Could you check a few things on this model? Use its own coordinates, in mm. Face numbers are marked on the shaded views. A direction names the side the tool comes from. Give positions to 0.01 mm unless a question says otherwise; leave off trailing zeros. Order: outer loops, then holes, each group sorted by start corner. A loop starts at its lowest first (then second) coordinate and runs counter-clockwise, first axis right, second up. Notation, with made-up numbers: (77.5, -11.5) - (98.5, -11.5) arc R28 ccw to (98.5, 23.5) - close; hole circle Ø11 at (41, -2). An arc over 180 degrees is marked (long way). Put each result on its own line as item: value.
from build123d import *

# Parameters (mm, degrees)
SKETCH1_W           = 100
SKETCH1_H           = 50
BOSS_EXTRUDE1_DEPTH = 15
SKETCH2_W           = 100
SKETCH2_H           = 65
BOSS_EXTRUDE2_DEPTH = 46
CUT_EXTRUDE1_DEPTH  = 47
CUT_EXTRUDE2_DEPTH  = 39
CUT_EXTRUDE3_DEPTH  = 26
FILLET1_R           = 15
SKETCH6_R           = 5
CUT_EXTRUDE4_DEPTH  = 75
SKETCH7_R           = 6
CUT_EXTRUDE5_DEPTH  = 26


with BuildPart() as part:
    # Sketch1 → Boss-Extrude1 (new body)
    with BuildSketch(Plane(origin=(0, 0, 0), x_dir=(1, 0, 0), z_dir=(0, 1, 0))):
        with Locations((0, -25)):
            Rectangle(SKETCH1_W, SKETCH1_H)
    extrude(amount=BOSS_EXTRUDE1_DEPTH)

    # Sketch2 → Boss-Extrude2 (add)
    with BuildSketch(Plane.XY):
        with Locations((0, 32.5)):
            Rectangle(SKETCH2_W, SKETCH2_H)
    extrude(amount=BOSS_EXTRUDE2_DEPTH)

    # Sketch3 → Cut-Extrude1 (cut, through all)
    with BuildSketch(Plane.XY.offset(46)):
        with BuildLine():
            Line((-12, 65), (-12, 40))
            ThreePointArc((-12, 40), (-8.485281374, 31.514718626), (0, 28))
            ThreePointArc((0, 28), (8.485281374, 31.514718626), (12, 40))
            Line((12, 40), (12, 65))
            Line((12, 65), (-12, 65))
        make_face()
    extrude(amount=-CUT_EXTRUDE1_DEPTH, mode=Mode.SUBTRACT)

    # Sketch4 → Cut-Extrude2 (cut, through all)
    with BuildSketch(Plane(origin=(-12, 0, 0), x_dir=(0, 0, -1), z_dir=(1, 0, 0))):
        Polygon((-31, 65), (-46, 50), (-46, 65), align=None)
    cut_extrude2 = extrude(amount=-CUT_EXTRUDE2_DEPTH, mode=Mode.SUBTRACT)

    # Mirror1: Cut-Extrude2 across plane
    add(cut_extrude2.mirror(Plane(origin=(0, 0, 0), x_dir=(0, 0, 1), z_dir=(1, 0, 0))), mode=Mode.SUBTRACT)

    # Sketch5 → Cut-Extrude3 (cut)
    with BuildSketch(Plane.ZY.offset(50)):
        Polygon((15, 65), (15, 15), (46, 15), (46, 50), (31, 65), align=None)
    cut_extrude3 = extrude(amount=-CUT_EXTRUDE3_DEPTH, mode=Mode.SUBTRACT)

    # Mirror2: Cut-Extrude3 across plane
    add(cut_extrude3.mirror(Plane(origin=(0, 0, 0), x_dir=(0, 0, 1), z_dir=(1, 0, 0))), mode=Mode.SUBTRACT)

    # Fillet1
    fillet1_edges = [part.edges().sort_by_distance(p)[0] for p in [
        (-50, 65, 7.5),
        (50, 7.5, 50),
        (-50, 7.5, 50),
        (50, 65, 7.5),
    ]]
    fillet(fillet1_edges, radius=FILLET1_R)

    # Sketch6 → Cut-Extrude4 (cut, through all)
    with BuildSketch(Plane(origin=(24, 0, 0), x_dir=(0, 0, -1), z_dir=(1, 0, 0))):
        with Locations((-31, 40)):
            Circle(SKETCH6_R)
    extrude(amount=-CUT_EXTRUDE4_DEPTH, mode=Mode.SUBTRACT)

    # Sketch7 → Cut-Extrude5 (cut)
    with BuildSketch(Plane(origin=(0, 15, 0), x_dir=(1, 0, 0), z_dir=(0, 1, 0))):
        with Locations((-35, -35)):
            Circle(SKETCH7_R)
    cut_extrude5 = extrude(amount=-CUT_EXTRUDE5_DEPTH, mode=Mode.SUBTRACT)

    # Mirror3: Cut-Extrude5 across plane
    add(cut_extrude5.mirror(Plane(origin=(0, 0, 0), x_dir=(0, 0, 1), z_dir=(1, 0, 0))), mode=Mode.SUBTRACT)


solid = part.part
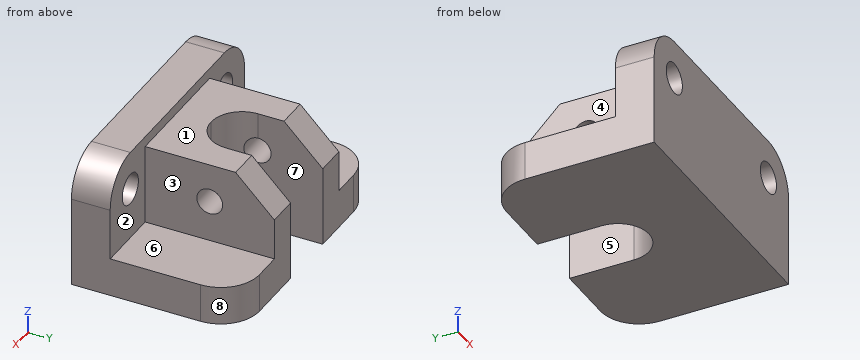
1) Suppose I cut it at D-D, the plane x = 6.5. List the corners of the cut face in (y, z) for me, and give its area (3 significant figures).
Filled in:
outline: (0, 0) - (29.91, 0) - (29.91, 46) - (15, 46) - (15, 50) - (0, 50) - close
area: 1,440 mm^2
2) Which directions (+Z, -Z, +X, -X, +Y, -Y) give clear straight access to the entire face, cutting with the end or side of a thin tool? Please do the marked faces 1, 2, 3 and 4.
Filled in:
face 1: +Z, +X, -X, +Y
face 2: +Z, +Y
face 3: +Z, +X, +Y
face 4: +Z, -X, +Y
3) I'm going to push flat-ended pins straight in: pin 1 (7.5 mm diameter, centred on y = 49.5, z = 28, fed in from +X); pin 2 (7.5 mm diameter, centred on y = 53, z = 25.5, fed in from -X); pin 3 (6 mm diameter, centred on x = -1.5, y = 18.5, fed in from +Z). Where does each tip first touch, or does it pass through?
Filled in:
pin 1: stops at x = 24
pin 2: stops at x = -24
pin 3: stops at z = 46
4) Suppose I cut it at A-A, the plane y = 13. List the corners of the cut face in (x, z) for me.
Filled in:
outline: (-50, 0) - (50, 0) - (50, 35) arc R15 ccw to (35, 50) - (-35, 50) arc R15 ccw to (-50, 35) - close; hole circle Ø12 at (-35, 35); hole circle Ø12 at (35, 35)
5) Suppose I cut it at C-C, the plane z = 23. List the corners of the cut face in (x, y) for me.
Filled in:
outline: (-50, 0) - (50, 0) - (50, 15) - (24, 15) - (24, 65) - (12, 65) - (12, 40) arc R12 cw to (-12, 40) - (-12, 65) - (-24, 65) - (-24, 15) - (-50, 15) - close
6) If I drill on line 1 (X direction, y = 6.5, z = 35); line 2 (Y direction, x = 20, z = 31); line 3 (Z direction, x = -35, y = 8.75), over which ranges is the centre line in solid material (lowest first)? Write a range as [from, to].
Filled in:
line 1: x = [-50, -41], [-29, 29], [41, 50]
line 2: y = [0, 35], [45, 65]
line 3: z = [0, 29], [41, 50]
7) Suppose I cut it at B-B, the plane y = 56. List the corners of the cut face in (x, z) for me.
Filled in:
outline: (-48.75, 0) - (-12, 0) - (-12, 40) - (-24, 40) - (-24, 15) - (-48.75, 15) - close; (12, 0) - (48.75, 0) - (48.75, 15) - (24, 15) - (24, 40) - (12, 40) - close
8) We'd pull the mould along X, two halves only. Please class the marked faces 5, 6, 7 and 8: pulls with the +X half, pulls with the -X half, needs draft (parallel to the pull), parting line crosses it, or undercut.
Filled in:
face 5: undercut
face 6: needs draft
face 7: undercut
face 8: pulls with the +X half
